Source: CAD feature listing. Evaluate the final solid. Frame: model axes, mm. Face numbers are marked on the shaded views. A direction names the side the tool comes from. Give positions to 0.01 mm unless a question says otherwise; leave off trailing zeros. Loops run counter-clockwise (first coordinate to the right, second up) from the corner with the lowest first, then second, coordinate; pieces in that order, holes last. Notation, with made-up numbers: (61.5, 45) -> (65.5, 45) arc R23 ccw to (65.5, 66) -> close; hole circle Ø2 at (36.5, 41.5). An arc over 180 degrees is marked (long way). Answer as a JSON object with one key per item and string values. Group by question number.
from build123d import *

# Parameters (mm, degrees)
F0_R     = 24
F0_R_2   = 12.7
F1_DEPTH = 24
F0_R_3   = 26
F2_DEPTH = 4
F3_START = 20
F3_DEPTH = 4
F4_SIZE  = 1.99999


# Not quite as in the source:
# - a fillet or chamfer is up to 0.001 mm smaller than in the source, because OpenCascade refuses the exact size


with BuildPart() as f1:
    # F0 (on Top) → F1 (new body)
    with BuildSketch(Plane.XY):
        Circle(F0_R)
        Circle(F0_R_2, mode=Mode.SUBTRACT)
    extrude(amount=F1_DEPTH)

    # F0 (on Top) → F2 (join)
    with BuildSketch(Plane.XY):
        Circle(F0_R_3)
        Circle(F0_R, mode=Mode.SUBTRACT)
    extrude(amount=F2_DEPTH)

    # F0 (on Top) → F3 (join)
    with BuildSketch(Plane.XY.offset(F3_START)):
        Circle(F0_R_3)
        Circle(F0_R, mode=Mode.SUBTRACT)
    extrude(amount=F3_DEPTH)

    # F4 (size 2 in the source; OpenCascade refuses exactly that, so slightly less here)
    f4_edges = [f1.edges().sort_by_distance(p)[0] for p in [
        (-26, 0, 20),
        (-26, 0, 24),
        (-26, 0, 4),
        (-26, 0, 0),
        (-12.7, 0, 0),
        (12.7, 0, 12),
        (-12.7, 0, 24),
    ]]
    chamfer(f4_edges, length=F4_SIZE)


solid = f1.part
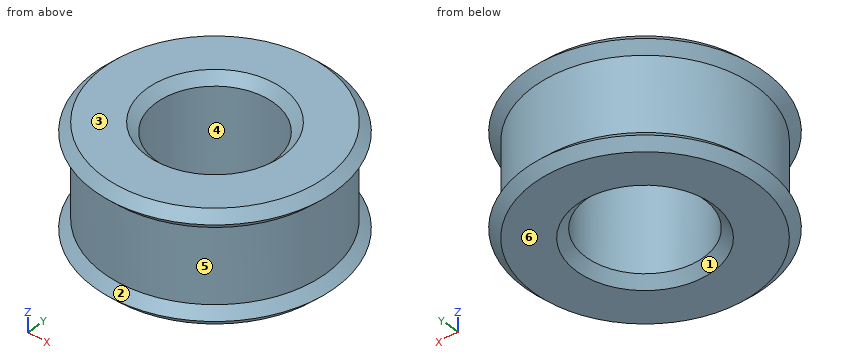
(1) Material intervals for line 1 (Y direction, x = 0, z = 17.5); line 2 (Y direction, x = 10, z = 14); line 3 (X direction, y = 11.5, z = 2.5), sorted ascending. Write a range as from..to.
(2) Access query for the marked faces 5 and 6. Directions: +Z, -Z, +X, -X, +Y, -Y. A direction counts if a zero-diameter tool reaches every point of the face in a straight line with its end or side. Return the directions, or none.
(3) Mould query, pull axis Y, two halves, no side actions, for the marked faces 1, 2, 3 and 4. Classes: pulls with the +Y half, pulls with the -Y half, needs draft (parallel to the pull), parting line crosses it, or undercut.
(4) First-contact query: pin 1 (3 mm diameter, centred on x = 13, z = 11.5, fed in from +Y); pin 2 (1.5 mm diameter, centred on x = -11, z = 12.5, fed in from -Y); pin 3 (6 mm diameter, centred on x = 3, y = -6, fed in from +Z); pin 4 (12 mm diameter, centred on y = 8.5, z = 10.5, fed in from -X). Flat tips, straight axial feed; report the tip coordinate or a pass-through.
(5) Section query C-C on z = 15. Return the cut outline in (x, y), plus the area to 3 significant figures.
Result:
{
 "1": {"line 1": "-24..-12.7, 12.7..24", "line 2": "-21.82..-7.83, 7.83..21.82", "line 3": "-22.76..-5.39, 5.39..22.76"},
 "2": {"face 5": "none", "face 6": "-Z, +X, -X, +Y, -Y"},
 "3": {"face 1": "undercut", "face 2": "parting line crosses it", "face 3": "needs draft", "face 4": "undercut"},
 "4": {"pin 1": "y = 21.07", "pin 2": "y = -21.7", "pin 3": "through", "pin 4": "x = -23.87"},
 "5": {"outline": "circle Ø48 at (0, 0); hole circle Ø25.4 at (0, 0)", "area": "1,300 mm²"}
}
